```python
from build123d import *

# Parameters (mm, degrees)
SKETCH1_R           = 22.225
BOSS_EXTRUDE1_DEPTH = 25.4
SKETCH2_R           = 25.4
SKETCH2_R_2         = 10.9140625
BOSS_EXTRUDE2_DEPTH = 12.7
SKETCH3_R           = 25.4
SKETCH3_R_2         = 12.7
CUT_EXTRUDE1_DEPTH  = 12.7
SKETCH5_R           = 27.051
SKETCH5_R_2         = 25.4
BOSS_EXTRUDE3_DEPTH = 2.54
SKETCH6_R           = 25.4
SKETCH6_R_2         = 23.749
CUT_EXTRUDE3_DEPTH  = 2.54


with BuildPart() as part:
    # Sketch1 → Boss-Extrude1 (new body)
    with BuildSketch(Plane(origin=(0, 0, 0), x_dir=(0, 0, -1), z_dir=(1, 0, 0))):
        Circle(SKETCH1_R)
        with BuildLine():
            Line((-1.5875, 6.148361062), (-1.5875, 7.9375))
            Line((-1.5875, 7.9375), (1.5875, 7.9375))
            Line((1.5875, 7.9375), (1.5875, 6.148361062))
            ThreePointArc((1.5875, 6.148361062), (5.020115786, 3.888564967), (6.35, 0))
            ThreePointArc((6.35, 0), (-3.888564967, -5.020115786), (-1.5875, 6.148361062))
        make_face(mode=Mode.SUBTRACT)
    extrude(amount=BOSS_EXTRUDE1_DEPTH)

    # Sketch2 → Boss-Extrude2 (add)
    with BuildSketch(Plane.ZY):
        Circle(SKETCH2_R)
        Circle(SKETCH2_R_2, mode=Mode.SUBTRACT)
    extrude(amount=-BOSS_EXTRUDE2_DEPTH)

    # Sketch3 → Cut-Extrude1 (cut)
    with BuildSketch(Plane(origin=(25.4, 0, 0), x_dir=(0, 0, -1), z_dir=(1, 0, 0))):
        Circle(SKETCH3_R)
        Circle(SKETCH3_R_2, mode=Mode.SUBTRACT)
    extrude(amount=-CUT_EXTRUDE1_DEPTH, mode=Mode.SUBTRACT)

    # Sketch5 → Boss-Extrude3 (add)
    with BuildSketch(Plane.ZY):
        Circle(SKETCH5_R)
        Circle(SKETCH5_R_2, mode=Mode.SUBTRACT)
    extrude(amount=-BOSS_EXTRUDE3_DEPTH)

    # Sketch6 → Cut-Extrude3 (cut)
    with BuildSketch(Plane(origin=(12.7, 0, 0), x_dir=(0, 0, -1), z_dir=(1, 0, 0))):
        Circle(SKETCH6_R)
        Circle(SKETCH6_R_2, mode=Mode.SUBTRACT)
    extrude(amount=-CUT_EXTRUDE3_DEPTH, mode=Mode.SUBTRACT)


solid = part.part
```
Check sheet for the modelled part. Datum: model origin and axes. Units: mm. A direction names the side the tool comes from. Give positions to 0.01 mm unless a question says otherwise; leave off trailing zeros. Write each loop counter-clockwise with the first axis right and the second up, starting at its lowest first coordinate (ties: lowest second). Pieces come first, ordered by that corner, then holes.
Item 1: Cross-section at B-B (y = 5). Enter the section's corners in (x, z).
Item 2: Access from +Z, -Z, +X, -X, +Y, -Y to the whole of each face (thin tool, end or side, straight path). Record for faces 1 (the face through (0, -6, 6)), 2 (the face through (12.7, -10, 10)), 3 (the face through (13, 7, -1.588)).
Item 3: Gauge pin test, flat ends, axial feed: pin 1 (1.5 mm diameter, centred on x = 10.5, y = 19.5, fed in from -Z); pin 2 (5 mm diameter, centred on x = 16, z = -21.5, fed in from -Y) (3 decimals); pin 3 (5 mm diameter, centred on x = 14, y = -11.5, fed in from +Z); pin 4 (10 mm diameter, centred on x = 15, y = 16, fed in from -Z). Record the tip position at first contact, or that the pin passes through.
Item 4: Scan lines: L1, parallel to Y at x = 19, z = 0; L2, parallel to Y at x = 7.5, z = 0; L3, parallel to X at y = 18, z = -10.5. Record each from-to range of solid material in increasing order.
Item 5: Cross-section at A-A (z = 0). Enter the section's corners in (x, y).
Item 6: Cross-section at C-C (x = 16.75). Enter the section's corners in (y, z), and give its area (3 significant figures).
Item 7: Cross-section at D-D (z = 17). Enter the section's corners in (x, y), and give its area (3 significant figures).
Item 8: Draft check along Z on faces 4 (the face through (13, 7.938, 0)), 5 (the face through (25.4, 6, -3)), 6 (the face through (11.448, 7.134, -22.652)). Enter one of: released by +Z, released by -Z, zero draft, split by the parting line, or undercut.
Report:
1. outline: (0, -26.58) - (2.54, -26.58) - (2.54, -24.9) - (10.16, -24.9) - (10.16, -23.22) - (12.7, -23.22) - (12.7, -11.67) - (25.4, -11.67) - (25.4, -3.91) - (0, -3.91) - close; (0, 3.91) - (25.4, 3.91) - (25.4, 11.67) - (12.7, 11.67) - (12.7, 23.22) - (10.16, 23.22) - (10.16, 24.9) - (2.54, 24.9) - (2.54, 26.58) - (0, 26.58) - close
2. face 1: +Z, -Z, -X, +Y, -Y
2. face 2: +X
2. face 3: +X, -X
3. pin 1: stops at z = -17.05
3. pin 2: passes through
3. pin 3: stops at z = 21.82
3. pin 4: stops at z = -20.75
4. L1: y = -12.7 to -6.35, 7.94 to 12.7
4. L2: y = -25.4 to -6.35, 7.94 to 25.4
4. L3: x = 0 to 12.7
5. outline: (0, -27.05) - (2.54, -27.05) - (2.54, -25.4) - (10.16, -25.4) - (10.16, -23.75) - (12.7, -23.75) - (12.7, -12.7) - (25.4, -12.7) - (25.4, -6.35) - (0, -6.35) - close; (0, 7.94) - (25.4, 7.94) - (25.4, 12.7) - (12.7, 12.7) - (12.7, 23.75) - (10.16, 23.75) - (10.16, 25.4) - (2.54, 25.4) - (2.54, 27.05) - (0, 27.05) - close
6. outline: circle Ø25.4 at (0, 0); hole (6.15, -1.59) - (7.94, -1.59) - (7.94, 1.59) - (6.15, 1.59) arc R6.35 ccw (long way) to start
6. area: 375 mm2
7. outline: (0, -21.04) - (2.54, -21.04) - (2.54, -18.87) - (10.16, -18.87) - (10.16, -16.58) - (12.7, -16.58) - (12.7, 16.58) - (10.16, 16.58) - (10.16, 18.87) - (2.54, 18.87) - (2.54, 21.04) - (0, 21.04) - close
7. area: 479 mm2
8. face 4: undercut
8. face 5: zero draft
8. face 6: split by the parting line
